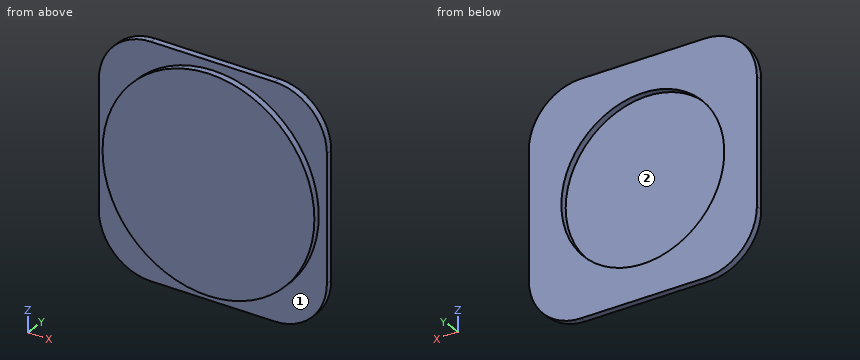
from build123d import *

# Parameters (mm, degrees)
SKETCH1_W           = 70
SKETCH1_H           = 70
SKETCH1_R           = 25
BOSS_EXTRUDE1_DEPTH = 2
FILLET1_R           = 16
SKETCH2_R           = 32.5
BOSS_EXTRUDE2_DEPTH = 2


with BuildPart() as part:
    # Sketch1 → Boss-Extrude1 (new body)
    with BuildSketch(Plane(origin=(0, 0, 0), x_dir=(1, 0, 0), z_dir=(0, 1, 0))):
        Rectangle(SKETCH1_W, SKETCH1_H)
        Circle(SKETCH1_R, mode=Mode.SUBTRACT)
    extrude(amount=BOSS_EXTRUDE1_DEPTH)

    # Fillet1
    fillet1_edges = [part.edges().sort_by_distance(p)[0] for p in [
        (35, 1, 35),
        (-35, 1, 35),
        (-35, 1, -35),
        (35, 1, -35),
    ]]
    fillet(fillet1_edges, radius=FILLET1_R)

    # Sketch2 → Boss-Extrude2 (add)
    with BuildSketch(Plane.XZ):
        Circle(SKETCH2_R)
    extrude(amount=BOSS_EXTRUDE2_DEPTH)


solid = part.part
Here's how the part is built. I have some questions about the finished solid (model axes, mm). Face numbers are marked on the shaded views. Coordinates: 2 decimals unless noted, no trailing zeros. Write each loop counter-clockwise with the first axis right and the second up, starting at its lowest first coordinate (ties: lowest second). Pieces come first, ordered by that corner, then holes.
1) If we section it at B-B (x = 0): List the corners of the cut face in (y, z) for me, plus the area to 3 significant figures.
Filled in:
outline: (-2, -32.5) - (0, -32.5) - (0, -35) - (2, -35) - (2, -25) - (0, -25) - (0, 25) - (2, 25) - (2, 35) - (0, 35) - (0, 32.5) - (-2, 32.5) - close
area: 170 mm2
2) If I drill on line 1 (Z direction, x = 0, y = 0.4); line 2 (Y direction, x = -18.5, z = 29), over which ranges is the centre line in solid material (lowest first)?
Filled in:
line 1: z = -35 to -25, 25 to 35
line 2: y = 0 to 2
3) If we section it at C-C (z = 0): List the corners of the cut face in (x, y) for me, plus the area to 3 significant figures.
Filled in:
outline: (-35, 0) - (-32.5, 0) - (-32.5, -2) - (32.5, -2) - (32.5, 0) - (35, 0) - (35, 2) - (25, 2) - (25, 0) - (-25, 0) - (-25, 2) - (-35, 2) - close
area: 170 mm2
4) Thinking about a two-plate mould opening in Z: for the marked faces 1 and 2, which applies, +Z half, -Z half, draft (parallel to the pull), parting line (faces both ways), or undercut?
Filled in:
face 1: draft
face 2: undercut
5) I'm going to push flat-ended pins straight in: pin 1 (8 mm diameter, centred on x = -12.5, z = 0, fed in from +Y); pin 2 (1.5 mm diameter, centred on x = -23.5, z = 26.5, fed in from -Y). Where does each tip first touch, or does it pass through?
Filled in:
pin 1: stops at y = 0
pin 2: stops at y = 0
6) If we section it at A-A (y = 0.65): List the corners of the cut face in (x, z) for me.
Filled in:
outline: (-35, -19) arc R16 ccw to (-19, -35) - (19, -35) arc R16 ccw to (35, -19) - (35, 19) arc R16 ccw to (19, 35) - (-19, 35) arc R16 ccw to (-35, 19) - close; hole circle Ø50 at (0, 0)
